Print and shaded views of the part. All mm, measured from the part's lowest x, y and z. Round coordinates to 2 decimals unless told otherwise and drop trailing zeros. Loops run counter-clockwise (first coordinate to the right, second up) from the corner with the lowest first, then second, coordinate; pieces in that order, holes last. Notation, with made-up numbers: (4, 25) - (34, 25) arc R32 ccw to (34, 64) - close; hole circle Ø8 at (70.25, 85.5). An arc over 180 degrees is marked (long way). Answer as a JSON object with one key per item and string values.
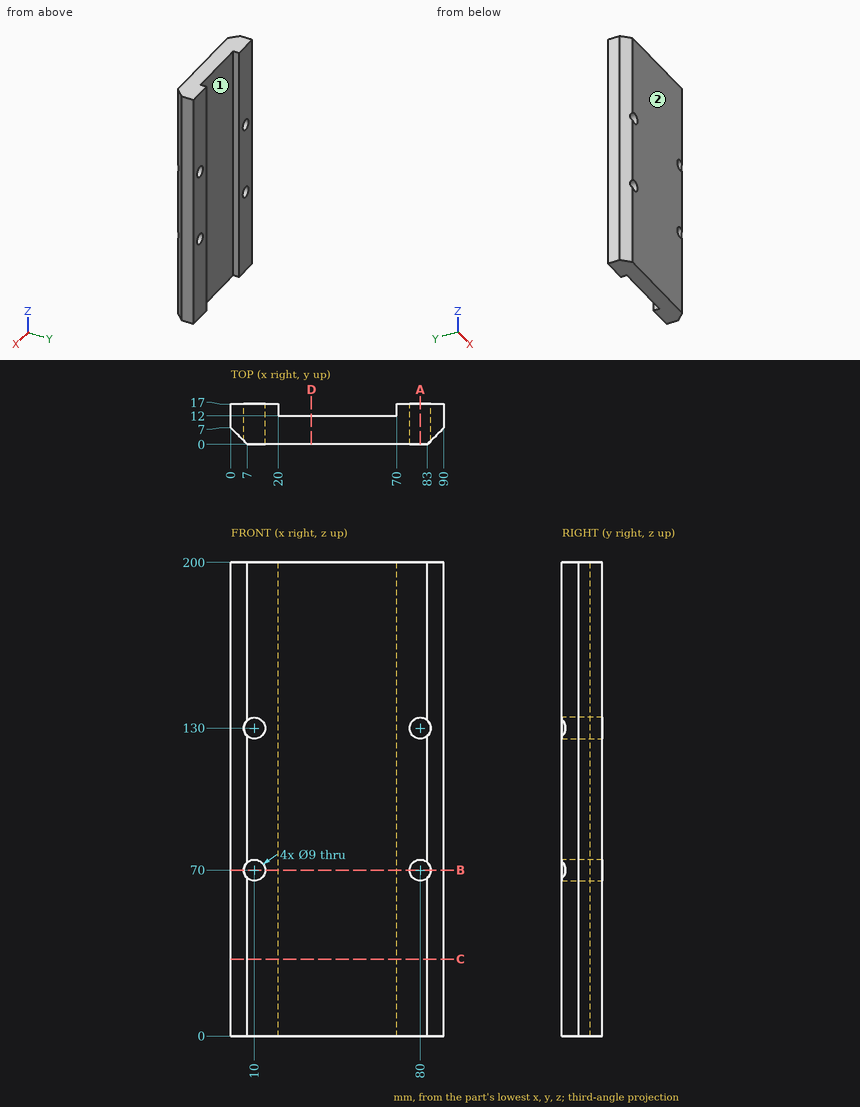
1) Drop a flat-ended pin along its axis: P1, Ø4, axis at x = 66.5, z = 65, coming from the +Y side. Give the stop position or say it passes through.
Values follow:
{"P1": "y = 12"}
2) Slice it at C-C on z = 32.5. List the corners of the cut face in (x, y), then the cut area to 3 significant figures.
Values follow:
{"outline": "(0, 7) - (7, 0) - (83, 0) - (90, 7) - (90, 17) - (70, 17) - (70, 12) - (20, 12) - (20, 17) - (0, 17) - close", "area": "1,230 mm²"}
3) Two-plate mould, pull along X, no slides. Class the marked faces 1 and 2: pulls with the +X half, pulls with the -X half, needs draft (parallel to the pull), parting line crosses it, or undercut.
Values follow:
{"face 1": "undercut", "face 2": "needs draft"}
4) Probe probe 1 along Z at (x, y) = (10, 12.5); probe 2 along X at (y, z) = (7.5, 70); probe 3 along X at (y, z) = (12.75, 70). List the from-to ranges inside material, lowest first.
Values follow:
{"probe 1": "0 to 65.5, 74.5 to 125.5, 134.5 to 200", "probe 2": "0 to 5.5, 14.5 to 75.5, 84.5 to 90", "probe 3": "0 to 5.5, 14.5 to 20, 70 to 75.5, 84.5 to 90"}
5) Slice it at D-D on x = 34. List the corners of the cut face in (y, z), then the cut area to 3 significant figures.
Values follow:
{"outline": "(0, 0) - (12, 0) - (12, 200) - (0, 200) - close", "area": "2,400 mm²"}
6) Slice it at A-A on x = 80. List the corners of the cut face in (y, z).
Values follow:
{"outline": "(0, 0) - (17, 0) - (17, 65.5) - (0, 65.5) - close; (0, 74.5) - (17, 74.5) - (17, 125.5) - (0, 125.5) - close; (0, 134.5) - (17, 134.5) - (17, 200) - (0, 200) - close"}
7) Slice it at B-B on z = 70. List the corners of the cut face in (x, y).
Values follow:
{"outline": "(0, 7) - (5.5, 1.5) - (5.5, 17) - (0, 17) - close; (14.5, 0) - (75.5, 0) - (75.5, 17) - (70, 17) - (70, 12) - (20, 12) - (20, 17) - (14.5, 17) - close; (84.5, 1.5) - (90, 7) - (90, 17) - (84.5, 17) - close"}
